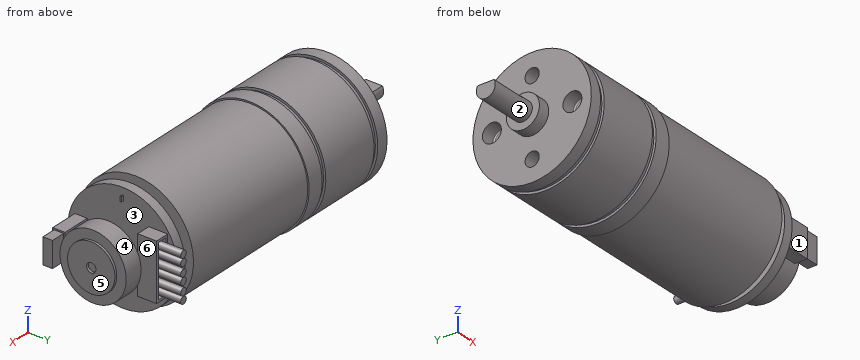
```python
from build123d import *

# Parameters (mm, degrees)
CROQUIS3_R               = 12.5
SALIENTE_EXTRUIR1_DEPTH  = 21
CROQUIS6_R               = 12.5
CROQUIS6_R_2             = 12
CORTAR_EXTRUIR3_DEPTH    = 1
CROQUIS7_R               = 12.5
CROQUIS7_R_2             = 12
CORTAR_EXTRUIR4_DEPTH    = 1
CROQUIS8_R               = 3.5
SALIENTE_EXTRUIR3_DEPTH  = 2.5
CROQUIS9_R               = 2
SALIENTE_EXTRUIR4_DEPTH  = 12.5
CROQUIS10_W              = 8
CROQUIS10_H              = 4
CORTAR_EXTRUIR5_DEPTH    = 5
CROQUIS11_R              = 1.5
CORTAR_EXTRUIR6_DEPTH    = 3
CROQUIS12_R              = 2
CORTAR_EXTRUIR7_DEPTH    = 3
CORTAR_EXTRUIR8_DEPTH    = 1.5
CORTAR_EXTRUIR9_DEPTH    = 1.5
REDONDEO1_R              = 0.25
CROQUIS16_W              = 1.05
CROQUIS16_H              = 0.3
SALIENTE_EXTRUIR5_DEPTH  = 4
CROQUIS17_R              = 4
SALIENTE_EXTRUIR6_DEPTH  = 0.75
SALIENTE_EXTRUIR7_START  = 0.75
CROQUIS18_R              = 3.5
SALIENTE_EXTRUIR7_DEPTH  = 0.75
CROQUIS19_R              = 11.6
SALIENTE_EXTRUIR8_DEPTH  = 2
CROQUIS20_R              = 1
SALIENTE_EXTRUIR9_DEPTH  = 4
CROQUIS21_R              = 7
SALIENTE_EXTRUIR10_DEPTH = 4
CROQUIS22_R              = 5
SALIENTE_EXTRUIR11_DEPTH = 0.5
CORTAR_EXTRUIR10_START   = -0.5
CROQUIS23_R              = 1
CORTAR_EXTRUIR10_DEPTH   = 0.5
SALIENTE_EXTRUIR12_DEPTH = 3
CORTAR_EXTRUIR11_DEPTH   = 3.5
CROQUIS26_R              = 0.75
SALIENTE_EXTRUIR13_DEPTH = 8
SALIENTE_EXTRUIR14_DEPTH = 6
CROQUIS28_W              = 5.4
CROQUIS28_H              = 2
SALIENTE_EXTRUIR15_DEPTH = 3


with BuildPart() as part:
    # Croquis1 → Revolución-Lámina1 (revolve)
    with BuildSketch(Plane.XY, mode=Mode.PRIVATE) as revoluci_n_l_mina1_sk:
        Polygon((0, 0), (0, 12.2), (30.8, 12.2), (30.8, 0), (20.8, 0), (20.8, 2.2), (10, 2.2), (10, 0), align=None)
    revolve(revoluci_n_l_mina1_sk.sketch.rotate(Axis((0, 0, 0), (1, 0, 0)), 90), axis=Axis((0, 0, 0), (1, 0, 0)))

    # Croquis3 → Saliente-Extruir1 (add)
    with BuildSketch(Plane.ZY):
        with Locations(Location((0, 0, 0), (0, 0, 180))):
            Circle(CROQUIS3_R)
    extrude(amount=SALIENTE_EXTRUIR1_DEPTH)

    # Croquis6 → Cortar-Extruir3 (cut)
    with BuildSketch(Plane(origin=(-17.5, 0, 0), x_dir=(0, 0, -1), z_dir=(1, 0, 0))):
        Circle(CROQUIS6_R)
        Circle(CROQUIS6_R_2, mode=Mode.SUBTRACT)
    extrude(amount=-CORTAR_EXTRUIR3_DEPTH, mode=Mode.SUBTRACT)

    # Croquis7 → Cortar-Extruir4 (cut)
    with BuildSketch(Plane(origin=(-3.5, 0, 0), x_dir=(0, 0, -1), z_dir=(1, 0, 0))):
        Circle(CROQUIS7_R)
        Circle(CROQUIS7_R_2, mode=Mode.SUBTRACT)
    extrude(amount=-CORTAR_EXTRUIR4_DEPTH, mode=Mode.SUBTRACT)

    # Croquis8 → Saliente-Extruir3 (add)
    with BuildSketch(Plane.ZY.offset(21)):
        Circle(CROQUIS8_R)
    extrude(amount=SALIENTE_EXTRUIR3_DEPTH)

    # Croquis9 → Saliente-Extruir4 (add)
    with BuildSketch(Plane.ZY.offset(21)):
        Circle(CROQUIS9_R)
    extrude(amount=SALIENTE_EXTRUIR4_DEPTH)

    # Croquis10 → Cortar-Extruir5 (cut)
    with BuildSketch(Plane.XY.offset(1)):
        with Locations((-29.5, 0)):
            Rectangle(CROQUIS10_W, CROQUIS10_H)
    extrude(amount=CORTAR_EXTRUIR5_DEPTH, mode=Mode.SUBTRACT)

    # Croquis11 → Cortar-Extruir6 (cut)
    with BuildSketch(Plane.ZY.offset(21)):
        with Locations((-8, 0)):
            Circle(CROQUIS11_R)
        with Locations((8, 0)):
            Circle(CROQUIS11_R)
    extrude(amount=-CORTAR_EXTRUIR6_DEPTH, mode=Mode.SUBTRACT)

    # Croquis12 → Cortar-Extruir7 (cut)
    with BuildSketch(Plane.ZY.offset(21)):
        with Locations((0, -8.5)):
            Circle(CROQUIS12_R)
        with Locations((0, 8.5)):
            Circle(CROQUIS12_R)
    extrude(amount=-CORTAR_EXTRUIR7_DEPTH, mode=Mode.SUBTRACT)

    # Croquis14 → Cortar-Extruir8 (cut)
    with BuildSketch(Plane.ZY.offset(18)):
        Polygon((-0.25, 8.25), (-0.25, 7.2), (0.25, 7.2), (0.25, 8.25), (1.3, 8.25), (1.3, 8.75), (0.25, 8.75), (0.25, 9.8), (-0.25, 9.8), (-0.25, 8.75), (-1.3, 8.75), (-1.3, 8.25), align=None)
    extrude(amount=-CORTAR_EXTRUIR8_DEPTH, mode=Mode.SUBTRACT)

    # Croquis15 → Cortar-Extruir9 (cut)
    with BuildSketch(Plane.ZY.offset(18)):
        Polygon((-0.25, -8.75), (-0.25, -9.8), (0.25, -9.8), (0.25, -8.75), (1.3, -8.75), (1.3, -8.25), (0.25, -8.25), (0.25, -7.2), (-0.25, -7.2), (-0.25, -8.25), (-1.3, -8.25), (-1.3, -8.75), align=None)
    extrude(amount=-CORTAR_EXTRUIR9_DEPTH, mode=Mode.SUBTRACT)

    # Redondeo1
    redondeo1_edges = [part.edges().sort_by_distance(p)[0] for p in [
        (-18, -8.5, -2),
        (-18, 8.5, -2),
    ]]
    fillet(redondeo1_edges, radius=REDONDEO1_R)

    # Croquis16 → Saliente-Extruir5 (add)
    with BuildSketch(Plane(origin=(30.8, 0, 0), x_dir=(0, 0, -1), z_dir=(1, 0, 0))):
        with Locations((-9.575, 0)):
            Rectangle(CROQUIS16_W, CROQUIS16_H)
        with Locations((8.525, 0)):
            Rectangle(CROQUIS16_W, CROQUIS16_H)
    extrude(amount=SALIENTE_EXTRUIR5_DEPTH)

    # Croquis17 → Saliente-Extruir6 (add)
    with BuildSketch(Plane(origin=(30.8, 0, 0), x_dir=(0, 0, -1), z_dir=(1, 0, 0))):
        Circle(CROQUIS17_R)
    extrude(amount=SALIENTE_EXTRUIR6_DEPTH)

    # Croquis18 → Saliente-Extruir7 (add)
    with BuildSketch(Plane(origin=(31.55, 0, 0), x_dir=(0, 0, -1), z_dir=(1, 0, 0)).offset(SALIENTE_EXTRUIR7_START)):
        with Locations(Location((0, 0, 0), (0, 0, 180))):
            Circle(CROQUIS18_R)
    extrude(amount=-SALIENTE_EXTRUIR7_DEPTH)

    # Croquis19 → Saliente-Extruir8 (add)
    with BuildSketch(Plane(origin=(32.3, 0, 0), x_dir=(0, 0, -1), z_dir=(1, 0, 0))):
        Circle(CROQUIS19_R)
    extrude(amount=SALIENTE_EXTRUIR8_DEPTH)

    # Croquis20 → Saliente-Extruir9 (add)
    with BuildSketch(Plane(origin=(34.3, 0, 0), x_dir=(0, 0, -1), z_dir=(1, 0, 0))):
        Circle(CROQUIS20_R)
    extrude(amount=SALIENTE_EXTRUIR9_DEPTH)

    # Croquis21 → Saliente-Extruir10 (add)
    with BuildSketch(Plane(origin=(38.3, 0, 0), x_dir=(0, 0, -1), z_dir=(1, 0, 0))):
        Circle(CROQUIS21_R)
    extrude(amount=SALIENTE_EXTRUIR10_DEPTH)

    # Croquis22 → Saliente-Extruir11 (add)
    with BuildSketch(Plane(origin=(42.3, 0, 0), x_dir=(0, 0, -1), z_dir=(1, 0, 0))):
        Circle(CROQUIS22_R)
    extrude(amount=SALIENTE_EXTRUIR11_DEPTH)

    # Croquis23 → Cortar-Extruir10 (cut)
    with BuildSketch(Plane(origin=(42.8, 0, 0), x_dir=(0, 0, -1), z_dir=(1, 0, 0)).offset(CORTAR_EXTRUIR10_START)):
        Circle(CROQUIS23_R)
    extrude(amount=CORTAR_EXTRUIR10_DEPTH, mode=Mode.SUBTRACT)

    # Croquis24 → Saliente-Extruir12 (add)
    with BuildSketch(Plane(origin=(34.3, 0, 0), x_dir=(0, 0, -1), z_dir=(1, 0, 0))):
        Polygon((0, 9.5), (6, 9.5), (6, 5.5), (-6, 5.5), (-6, 9.5), align=None)
    extrude(amount=SALIENTE_EXTRUIR12_DEPTH)

    # Croquis25 → Cortar-Extruir11 (cut)
    with BuildSketch(Plane(origin=(0, 9.5, 0), x_dir=(1, 0, 0), z_dir=(0, 1, 0))):
        Polygon((36.8, -5.5), (36.8, 5.5), (34.8, 5.5), (34.8, -5.5), (35.8, -5.5), align=None)
    extrude(amount=-CORTAR_EXTRUIR11_DEPTH, mode=Mode.SUBTRACT)

    # Croquis26 → Saliente-Extruir13 (add)
    with BuildSketch(Plane(origin=(0, 6, 0), x_dir=(1, 0, 0), z_dir=(0, 1, 0))):
        with Locations(Location((35.8, -4.4, 0), (0, 0, 270))):
            Circle(CROQUIS26_R)
        with Locations(Location((35.8, -2.8, 0), (0, 0, 270))):
            Circle(CROQUIS26_R)
        with Locations(Location((35.8, -0.8, 0), (0, 0, 270))):
            Circle(CROQUIS26_R)
        with Locations(Location((35.8, 0.8, 0), (0, 0, 270))):
            Circle(CROQUIS26_R)
        with Locations(Location((35.8, 2.8, 0), (0, 0, 270))):
            Circle(CROQUIS26_R)
        with Locations(Location((35.8, 4.4, 0), (0, 0, 270))):
            Circle(CROQUIS26_R)
    extrude(amount=SALIENTE_EXTRUIR13_DEPTH)

    # Croquis27 → Saliente-Extruir14 (add)
    with BuildSketch(Plane(origin=(34.3, 0, 0), x_dir=(0, 0, -1), z_dir=(1, 0, 0))):
        Polygon((0, -10.1), (3, -10.1), (3, -7.5), (-3, -7.5), (-3, -10.1), align=None)
    extrude(amount=SALIENTE_EXTRUIR14_DEPTH)

    # Croquis28 → Saliente-Extruir15 (add)
    with BuildSketch(Plane(origin=(40.3, 0, 0), x_dir=(0, 0, -1), z_dir=(1, 0, 0))):
        with Locations((0, -8.8)):
            Rectangle(CROQUIS28_W, CROQUIS28_H)
    extrude(amount=SALIENTE_EXTRUIR15_DEPTH)


solid = part.part
```
Design review of the part built by this model. Coordinates are the model's own, in mm. Face numbers are marked on the shaded views. A direction names the side the tool comes from. Give positions to 0.01 mm unless a question says otherwise; leave off trailing zeros. Loops run counter-clockwise (first coordinate to the right, second up) from the corner with the lowest first, then second, coordinate; pieces in that order, holes last. Notation, with made-up numbers: M -40,89 L 14,89 A13 ccw 14,108 Z; hole C 67.5,67 d5. An arc over 180 degrees is marked long. Return JSON: item names as keys, results as strings. Group by question number.
Item 1: We need section C-C (x = -2.5). Give the boundary of the cut face in (y, z).
Item 2: Mouldability with a two-part tool opening along X and no side actions: class the marked faces 4, 5 and 6 as released by +X, released by -X, zero draft, split by the parting line, or undercut.
Item 3: We need section D-D (x = 22.5). Give the boundary of the cut face in (y, z), and give its area (3 significant figures).
Item 4: Insertion check: pin 1 Ø0.5 at (x, z) = (-17, 1) entering from +Y; pin 2 Ø2 at (y, z) = (-2, -9.5) entering from -X; pin 3 Ø12 at (y, z) = (0, 5.5) entering from -X; pin 4 Ø0.8 at (x, z) = (-17.5, -1) entering from -Y. Each pin has a flat end and moves straight along its axis. Give the tip position at first contact, or say it passes through.
Item 5: We need section B-B (x = 11). Give the boundary of the cut face in (y, z), and give its area (3 significant figures).
Item 6: Tool access review of the marked faces 1, 2 and 3: name each direction out of +Z, -Z, +X, -X, +Y, -Y from which nothing blocks a thin tool from reaching the whole face with its end or side.
Item 7: We need section A-A (x = 35.8). Give the number of separate pieces and of enclosed holes in the cut face, and give its area (3 significant figures).
Item 8: For probe 1 along X at (y, z) = (10.5, -4.5); probe 2 along X at (y, z) = (4.75, -3.75); probe 3 along X at (y, z) = (-5.5, -4.75), list the stretches that pass through material, from the lowest coordinate up.
Output:
{
 "1": {"outline": "C 0,0 d25"},
 "2": {"face 4": "zero draft", "face 5": "released by +X", "face 6": "undercut"},
 "3": {"outline": "C 0,0 d24.4", "area": "468 mm^2"},
 "4": {"pin 1": "stops at y = 12.48", "pin 2": "stops at x = -21", "pin 3": "stops at x = -33.5", "pin 4": "stops at y = -12.49"},
 "5": {"outline": "C 0,0 d24.4; hole C 0,0 d4.4", "area": "452 mm^2"},
 "6": {"face 1": "+Z, -Z, +X, -Y", "face 2": "-X", "face 3": "none"},
 "7": {"separate pieces": "3", "enclosed holes": "0", "area": "100 mm^2"},
 "8": {"probe 1": "x = -21 to 30.8, 32.3 to 34.3, 35.06 to 36.54", "probe 2": "x = -21 to 30.8, 32.3 to 34.3, 38.3 to 42.3", "probe 3": "x = -21 to 30.8, 32.3 to 34.3"}
}
